Input: part model. Units: mm. Frame: model coordinates. A direction names the side the tool comes from. Round coordinates to 2 decimals unless told otherwise and drop trailing zeros. Loops run counter-clockwise (first coordinate to the right, second up) from the corner with the lowest first, then second, coordinate; pieces in that order, holes last.
1) Ray query, line 1 along X through (y, z) = (9.75, 15.25); line 2 along X through (y, z) = (14.5, 14); line 3 along Y through (x, z) = (5.5, 11.75). Return the intervals inside material, ascending.
2) Access query for faces 1 (the face through (-2, -4, 10)), 2 (the face through (11, 0, 10)). Directions: +Z, -Z, +X, -X, +Y, -Y. A direction counts if a zero-diameter tool reaches every point of the face in a straight line with its end or side. Return the directions, or none.
3) First-contact query: pin 1 (10 mm diameter, centred on x = 11.5, z = 11.5, fed in from -Y); pin 2 (8 mm diameter, centred on x = 4, y = 10, fed in from +Z); pin 3 (5 mm diameter, centred on y = 11, z = 6, fed in from +X); pin 4 (3 mm diameter, centred on y = -2, z = 15, fed in from +X). Flat tips, straight axial feed; report the tip coordinate or a pass-through.
4) Section B-B, the plane x = 4. Return loops of the section in (y, z), and give its area (3 significant figures).
5) Draft query along X for faces 3 (the face through (-3, 10, 10)), 4 (the face through (0, 13, 10)), 5 (the face through (9, 7, 0)), 6 (the face through (12.14, 13.644, 9.86)). Return one class per face: pulls with the +X half, pulls with the -X half, needs draft (parallel to the pull), parting line crosses it, or undercut.
6) Section C-C, the plane y = 10. Return loops of the section in (x, z), and give its area (3 significant figures).
7) Section D-D, the plane y = -1.5. Return loops of the section in (x, z), and give its area (3 significant figures).
8) Section A-A, the plane z = 13.25. Return loops of the section in (x, y).
from build123d import *

# Parameters (mm, degrees)
ESQUISSE1_R          = 5
BASE_EXTRUSION_DEPTH = 20


with BuildPart() as part:
    # Esquisse1 → Base-Extrusion (new body)
    with BuildSketch(Plane.XY):
        Polygon((0, 0), (22, 0), (22, 3.574468085), (2, 24), (-3, 24), (-3, -4), (0, -4), align=None)
        with Locations((4, 10)):
            Circle(ESQUISSE1_R, mode=Mode.SUBTRACT)
    extrude(amount=BASE_EXTRUSION_DEPTH)


solid = part.part
Final values:
1. line 1: x = -3 to -0.99, 8.99 to 15.95
1. line 2: x = -3 to 1.82, 6.18 to 11.3
1. line 3: y = 0 to 5.23, 14.77 to 20.43
2. face 1: +Z, -Z, +X, -X, -Y
2. face 2: +Z, -Z, +X, -Y
3. pin 1: stops at y = 0
3. pin 2: passes through
3. pin 3: stops at x = 17.18
3. pin 4: stops at x = 0
4. outline: (0, 0) - (5, 0) - (5, 20) - (0, 20) - close; (15, 0) - (21.96, 0) - (21.96, 20) - (15, 20) - close
4. area: 239 mm2
5. face 3: pulls with the -X half
5. face 4: undercut
5. face 5: needs draft
5. face 6: pulls with the +X half
6. outline: (-3, 0) - (-1, 0) - (-1, 20) - (-3, 20) - close; (9, 0) - (15.71, 0) - (15.71, 20) - (9, 20) - close
6. area: 174 mm2
7. outline: (-3, 0) - (0, 0) - (0, 20) - (-3, 20) - close
7. area: 60.0 mm2
8. outline: (-3, -4) - (0, -4) - (0, 0) - (22, 0) - (22, 3.57) - (2, 24) - (-3, 24) - close; hole circle Ø10 at (4, 10)
